```python
from build123d import *

# Parameters (mm, degrees)
BOSS_EXTRUDE1_DEPTH = 3


with BuildPart() as part:
    # Sketch1 → Boss-Extrude1 (new body)
    with BuildSketch(Plane.XY):
        with BuildLine():
            Line((39.37, 34.29), (-39.37, 34.29))
            ThreePointArc((-39.37, 34.29), (-41.166051224, 33.546051224), (-41.91, 31.75))
            Line((-41.91, 31.75), (-41.91, -31.75))
            ThreePointArc((-41.91, -31.75), (-41.166051224, -33.546051224), (-39.37, -34.29))
            Line((-39.37, -34.29), (39.37, -34.29))
            ThreePointArc((39.37, -34.29), (41.166051224, -33.546051224), (41.91, -31.75))
            Line((41.91, -31.75), (41.91, 31.75))
            ThreePointArc((41.91, 31.75), (41.166051224, 33.546051224), (39.37, 34.29))
        make_face()
        with BuildLine():
            Line((-30.48, 25.4), (30.48, 25.4))
            ThreePointArc((30.48, 25.4), (32.276051224, 24.656051224), (33.02, 22.86))
            Line((33.02, 22.86), (33.02, -22.86))
            ThreePointArc((33.02, -22.86), (32.276051224, -24.656051224), (30.48, -25.4))
            Line((30.48, -25.4), (-30.48, -25.4))
            ThreePointArc((-30.48, -25.4), (-32.276051224, -24.656051224), (-33.02, -22.86))
            Line((-33.02, -22.86), (-33.02, 22.86))
            ThreePointArc((-33.02, 22.86), (-32.276051224, 24.656051224), (-30.48, 25.4))
        make_face(mode=Mode.SUBTRACT)
    extrude(amount=BOSS_EXTRUDE1_DEPTH)

    # Sketch3 → M2 Clearance Hole1 (revolve, cut)
    with BuildSketch(Plane(origin=(-39.033101712, 31.267063068, 3), x_dir=(0, -1, 0), z_dir=(1, 0, 0))):
        Polygon((0, 0), (0, 3.769032743), (1.2, 3.048), (1.2, 0), align=None)
    m2_clearance_hole1 = revolve(axis=Axis((-39.033101712, 31.267063068, 9.35), (0, 0, -1)), mode=Mode.SUBTRACT)

    # Mirror1: M2 Clearance Hole1 across plane
    add(m2_clearance_hole1.mirror(Plane.ZX), mode=Mode.SUBTRACT)

    # Mirror2: M2 Clearance Hole1 across plane
    add(m2_clearance_hole1.mirror(Plane(origin=(0, 0, 0), x_dir=(0, 0, 1), z_dir=(1, 0, 0))), mode=Mode.SUBTRACT)

    # Mirror2 copy 1 sketch → Mirror2 copy 1 (revolve, cut)
    with BuildSketch(Plane(origin=(39.033101712, -31.267063068, 3), x_dir=(0, 1, 0), z_dir=(-1, 0, 0))):
        Polygon((0, 0), (0, 3.769032743), (1.2, 3.048), (1.2, 0), align=None)
    revolve(axis=Axis((39.033101712, -31.267063068, 9.35), (0, 0, -1)), mode=Mode.SUBTRACT)


solid = part.part
```
Design review of the part built by this model. Coordinates are the model's own, in mm. A direction names the side the tool comes from. Round coordinates to 2 decimals unless told otherwise and drop trailing zeros. Write each loop counter-clockwise with the first axis right and the second up, starting at its lowest first coordinate (ties: lowest second). Pieces come first, ordered by that corner, then holes. Notation, with made-up numbers: (29.25, 16) -> (59.25, 16) arc R9 cw to (59.25, 32) -> close; hole circle Ø7 at (35, 25). An arc over 180 degrees is marked (long way). Write item = value, one per line. Start each with the question number.
1) Mouldability with a two-part tool opening along X and no side actions: class faces 1 (the face through (-1, -34.29, 1)), 2 (the face through (-37.97, 30.71, 1.52)), 3 (the face through (-41.91, 0, 1)) as +X half, -X half, draft (parallel to the pull), parting line (faces both ways), or undercut.
2) Tool access review of faces 4 (the face through (32.256, 24.676, 1.479)), 5 (the face through (1, 34.29, 1)): name each direction out of +Z, -Z, +X, -X, +Y, -Y from which nothing blocks a thin tool from reaching the whole face with its end or side.
3) Take a section at A-A, the plane y = -8.5. State the section outline as (x, z) points, plus the area to 3 significant figures.
4) Take a section at C-C, the plane z = 1.05. State the section outline as (x, y) points, plus the area to 3 significant figures.
5) Wall thickness on probe 1 along X at (y, z) = (-14, 2.3); probe 2 along Y at (x, z) = (27.5, 0.6); probe 3 along X at (y, z) = (-31, 0.65): over which ranges is each line inside the solid? List them lowest first. Write a range as from..to.
6) Take a section at B-B, the plane x = -6. State the section outline as (y, z) points, plus the area to 3 significant figures.
Results list:
q1.face_1 = draft
q1.face_2 = undercut
q1.face_3 = -X half
q2.face_4 = +Z, -Z
q2.face_5 = +Z, -Z, +X, -X, +Y
q3.outline = (-41.91, 0) -> (-33.02, 0) -> (-33.02, 3) -> (-41.91, 3) -> close; (33.02, 0) -> (41.91, 0) -> (41.91, 3) -> (33.02, 3) -> close
q3.area = 53.3 mm²
q4.outline = (-41.91, -31.75) arc R2.54 ccw to (-39.37, -34.29) -> (39.37, -34.29) arc R2.54 ccw to (41.91, -31.75) -> (41.91, 31.75) arc R2.54 ccw to (39.37, 34.29) -> (-39.37, 34.29) arc R2.54 ccw to (-41.91, 31.75) -> close; hole circle Ø2.4 at (-39.03, -31.27); hole circle Ø2.4 at (-39.03, 31.27); hole (-33.02, -22.86) arc R2.54 ccw to (-30.48, -25.4) -> (30.48, -25.4) arc R2.54 ccw to (33.02, -22.86) -> (33.02, 22.86) arc R2.54 ccw to (30.48, 25.4) -> (-30.48, 25.4) arc R2.54 ccw to (-33.02, 22.86) -> close; hole circle Ø2.4 at (39.03, -31.27); hole circle Ø2.4 at (39.03, 31.27)
q4.area = 2,380 mm²
q5.probe_1 = -41.91..-33.02, 33.02..41.91
q5.probe_2 = -34.29..-25.4, 25.4..34.29
q5.probe_3 = -41.91..-40.2, -37.86..37.86, 40.2..41.91
q6.outline = (-34.29, 0) -> (-25.4, 0) -> (-25.4, 3) -> (-34.29, 3) -> close; (25.4, 0) -> (34.29, 0) -> (34.29, 3) -> (25.4, 3) -> close
q6.area = 53.3 mm²
